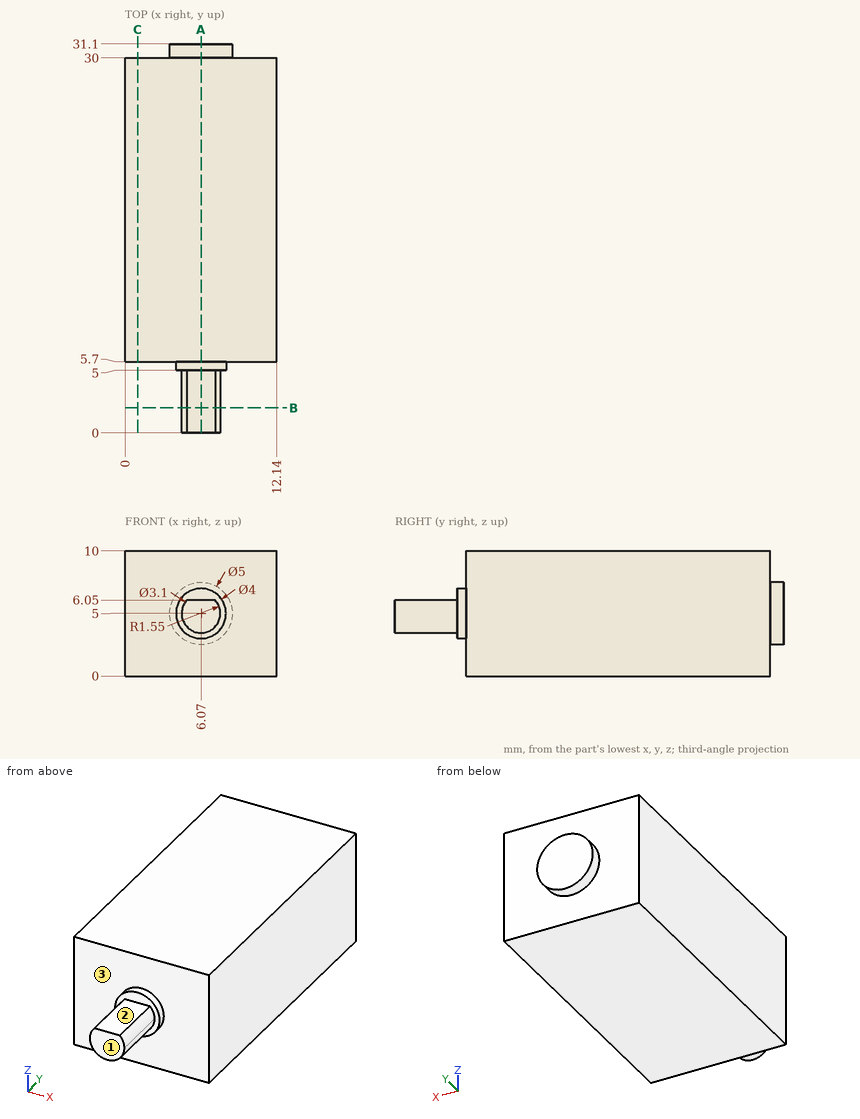
Check sheet for the drawn part. Datum: minimum x, y, z corner. Units: mm. A direction names the side the tool comes from. Give positions to 0.01 mm unless a question says otherwise; leave off trailing zeros. Order: outer loops, then holes, each group sorted by start corner. A loop starts at its lowest first (then second) coordinate and runs counter-clockwise, first axis right, second up. Notation, with made-up numbers: (-22, -28.5) -> (13, -28.5) arc R27 cw to (13, -12.5) -> close; hole circle Ø2 at (29, -16). An arc over 180 degrees is marked (long way). Return JSON: item names as keys, results as strings.
1. Cross-section at A-A, the plane x = 6.07. Record the cut outline in (y, z).
From the geometry:
{"outline": "(0, 3.45) -> (5, 3.45) -> (5, 3) -> (5.7, 3) -> (5.7, 0) -> (30, 0) -> (30, 2.5) -> (31.1, 2.5) -> (31.1, 7.5) -> (30, 7.5) -> (30, 10) -> (5.7, 10) -> (5.7, 7) -> (5, 7) -> (5, 6.05) -> (0, 6.05) -> close"}
2. Set-up check for the marked faces 1, 2 and 3: record each of +Z, -Z, +X, -X, +Y, -Y from which the full face is reachable in a straight line by a thin tool's end or side.
From the geometry:
{"face 1": "+Z, -Z, +X, -X, -Y", "face 2": "+Z, +X, -X, -Y", "face 3": "-Y"}
3. Cross-section at B-B, the plane y = 2. Record the cut outline in (x, z).
From the geometry:
{"outline": "(4.93, 6.05) arc R1.55 ccw (long way) to (7.62, 5) arc R1.55 ccw to (7.21, 6.05) -> close"}
4. Go/stop test with flat-tipped pins: P1, Ø5, axis at x = 6, y = 5.5, coming from the +Z side; P2, Ø2.5, axis at x = 5.5, y = 1.5, coming from the +Z side. Record where each tip stops, or that it passes through.
From the geometry:
{"P1": "z = 10", "P2": "z = 6.05"}
5. Material ranges on probe 1 along Y at (x, z) = (7.75, 9.25); probe 2 along Y at (x, z) = (7.5, 6.5); probe 3 along X at (y, z) = (2.5, 4), recorded low to high. Write a range as [from, to].
From the geometry:
{"probe 1": "[5.7, 30]", "probe 2": "[5.7, 31.1]", "probe 3": "[4.89, 7.25]"}
6. Cross-section at C-C, the plane x = 1. Record the cut outline in (y, z), plus the area to 3 significant figures.
From the geometry:
{"outline": "(5.7, 0) -> (30, 0) -> (30, 10) -> (5.7, 10) -> close", "area": "243 mm^2"}
